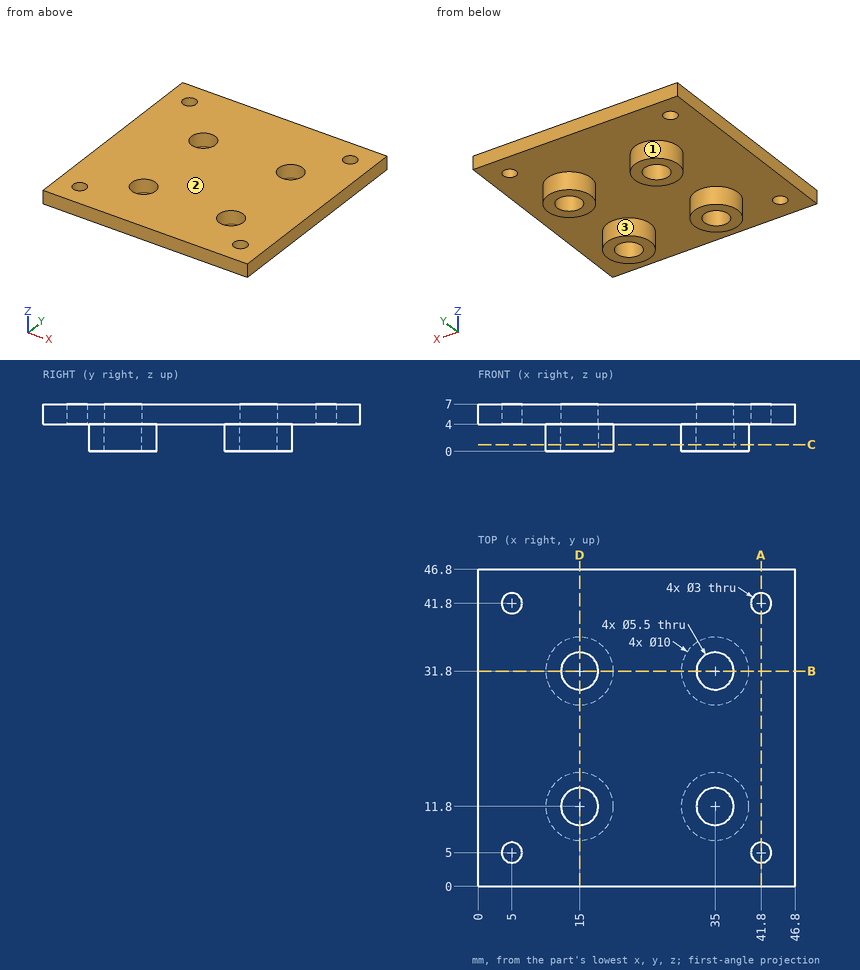
The figure shows three views and two pictorial views of one solid part (mm, origin at its lowest corner). Answer the questions. Round coordinates to 2 decimals unless told otherwise and drop trailing zeros. Loops run counter-clockwise (first coordinate to the right, second up) from the corner with the lowest first, then second, coordinate; pieces in that order, holes last. Notation, with made-up numbers: M 2.5,-9.75 L 58.5,-9.75 A17 ccw 58.5,1.25 Z; hole C -39,-21.75 d2. An arc over 180 degrees is marked long. Return JSON: item names as keys, results as strings.
Q1. Find section B-B, the plane y = 31.8. Determine the outline of the cut face in (x, z).
Results list:
{"outline": "M 0,4 L 10,4 L 10,0 L 12.25,0 L 12.25,7 L 0,7 Z; M 17.75,0 L 20,0 L 20,4 L 30,4 L 30,0 L 32.25,0 L 32.25,7 L 17.75,7 Z; M 37.75,0 L 40,0 L 40,4 L 46.8,4 L 46.8,7 L 37.75,7 Z"}
Q2. Find the intervals of material crossed by line 1 along X through (y, z) = (32, 5.25); line 2 along Y through (x, z) = (5, 6.25); line 3 along Y through (x, z) = (35, 1.2), in increasing order. Write a range as from..to.
Results list:
{"line 1": "x = 0..12.26, 17.74..32.26, 37.74..46.8", "line 2": "y = 0..3.5, 6.5..40.3, 43.3..46.8", "line 3": "y = 6.8..9.05, 14.55..16.8, 26.8..29.05, 34.55..36.8"}
Q3. Find section C-C, the plane z = 1. Determine the outline of the cut face in (x, y).
Results list:
{"outline": "C 15,11.8 d10; C 15,31.8 d10; C 35,11.8 d10; C 35,31.8 d10; hole C 15,11.8 d5.5; hole C 15,31.8 d5.5; hole C 35,11.8 d5.5; hole C 35,31.8 d5.5"}
Q4. The mould has two halves that part along X. Classify the marked faces 1, 2 and 3: released by +X, released by -X, zero draft, split by the parting line, or undercut.
Results list:
{"face 1": "undercut", "face 2": "zero draft", "face 3": "undercut"}
Q5. This flat-tipped pin is pushed along its axis until it touches: pin 1 Ø1.5 at (x, y) = (30, 23) entering from -Z. Where does it stop, or does it pass through?
Results list:
{"pin 1": "stops at z = 4"}
Q6. Find section A-A, the plane x = 41.8. Determine the outline of the cut face in (y, z), plus the area to 3 significant figures.
Results list:
{"outline": "M 0,4 L 3.5,4 L 3.5,7 L 0,7 Z; M 6.5,4 L 40.3,4 L 40.3,7 L 6.5,7 Z; M 43.3,4 L 46.8,4 L 46.8,7 L 43.3,7 Z", "area": "122 mm2"}
Q7. Find section D-D, the plane x = 15. Determine the outline of the cut face in (y, z).
Results list:
{"outline": "M 0,4 L 6.8,4 L 6.8,0 L 9.05,0 L 9.05,7 L 0,7 Z; M 14.55,0 L 16.8,0 L 16.8,4 L 26.8,4 L 26.8,0 L 29.05,0 L 29.05,7 L 14.55,7 Z; M 34.55,0 L 36.8,0 L 36.8,4 L 46.8,4 L 46.8,7 L 34.55,7 Z"}
